Can you work these out from the model? Positions are in its coordinate system, mm. Give positions to 0.01 mm unless a question says otherwise; leave off trailing zeros. Write each loop counter-clockwise with the first axis right and the second up, starting at its lowest first coordinate (ties: lowest second). Pieces come first, ordered by that corner, then holes. Notation, with made-up numbers: (37, 82.5) -> (90, 82.5) arc R21 ccw to (90, 119.5) -> close; hole circle Ø7 at (13, 66.5). An arc over 180 degrees is marked (long way). Answer as CSV lines item,"result". Start each with the question number.
1. If we section it at D-D on x = 22.5: Write out the boundary of the cut face in (y, z).
2. I'm going to push flat-ended pins straight in: P1, Ø3, axis at x = 22.5, y = 5, coming from the +Z side; P2, Ø4, axis at x = 35.5, z = -129, coming from the -Y side; P3, Ø1.4, axis at x = 37, y = 6.5, coming from the -Z side; P4, Ø5.5, axis at x = 36, z = -75.5, coming from the +Y side. Where does each tip first touch, or does it pass through?
3. I need wall thicknesses on line 1 (X direction, y = 5.5, z = -110); line 2 (X direction, y = 2, z = -56); line 3 (Y direction, x = 7.5, z = -44). Which ranges of each line are inside material? Lowest first, please. Write a range as [from, to].
4. If we section it at C-C on y = 5: Count the separate pieces of the cut face and the enclosed holes in it, plus the area to 3 significant figures.
5. If we section it at A-A on z = -82: Write out the boundary of the cut face in (x, y).
6. If we section it at B-B on x = 12: Write out the boundary of the cut face in (y, z), plus the area to 3 significant figures.
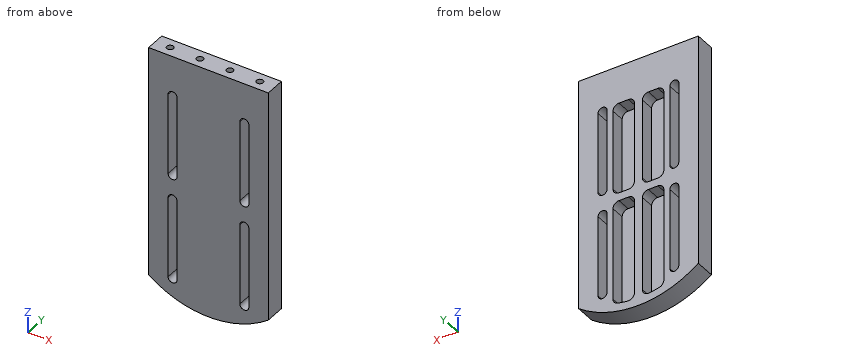
```python
from build123d import *

# Parameters (mm, degrees)
EXTRUDE_1_DEPTH     = 10
CUT_EXTRUDE_1_DEPTH = 7
EXTRUDE_2_REACH     = 173.532
SKETCH_3_W          = 10.75
SKETCH_3_H          = 4
FILLET_1_R          = 3
M4X0_71_D           = 3.3
M4X0_71_DEPTH       = 15
SKETCH_9_W          = 60
SKETCH_9_H          = 23.75
SKETCH_9_H_2        = 5
CUT_EXTRUDE_2_DEPTH = 10


with BuildPart() as part:
    # Эскиз1 → Бобышка-Вытянуть1 (new body)
    with BuildSketch(Plane(origin=(0, 0, 0), x_dir=(1, 0, 0), z_dir=(0, 1, 0))):
        with BuildLine():
            Line((0, 0), (0, 150.384470983))
            ThreePointArc((0, 150.384470983), (30, 160.384470983), (60, 150.384470983))
            Line((60, 150.384470983), (60, 0))
            Line((60, 0), (0, 0))
        make_face()
        with BuildLine():
            Line((14.25, 147.6), (14.25, 102))
            ThreePointArc((14.25, 102), (12, 99.75), (9.75, 102))
            Line((9.75, 102), (9.75, 147.6))
            ThreePointArc((9.75, 147.6), (12, 149.85), (14.25, 147.6))
        make_face(mode=Mode.SUBTRACT)
        with BuildLine():
            Line((50.25, 147.6), (50.25, 102))
            ThreePointArc((50.25, 102), (48, 99.75), (45.75, 102))
            Line((45.75, 102), (45.75, 147.6))
            ThreePointArc((45.75, 147.6), (48, 149.85), (50.25, 147.6))
        make_face(mode=Mode.SUBTRACT)
        with BuildLine():
            Line((14.25, 89.6), (14.25, 44))
            ThreePointArc((14.25, 44), (12, 41.75), (9.75, 44))
            Line((9.75, 44), (9.75, 89.6))
            ThreePointArc((9.75, 89.6), (12, 91.85), (14.25, 89.6))
        make_face(mode=Mode.SUBTRACT)
        with BuildLine():
            Line((45.75, 89.6), (45.75, 44))
            ThreePointArc((45.75, 44), (48, 41.75), (50.25, 44))
            Line((50.25, 44), (50.25, 89.6))
            ThreePointArc((50.25, 89.6), (48, 91.85), (45.75, 89.6))
        make_face(mode=Mode.SUBTRACT)
    extrude(amount=EXTRUDE_1_DEPTH)

    # Эскиз2 → Вырез-Вытянуть1 (cut)
    with BuildSketch(Plane(origin=(0, 10, 0), x_dir=(1, 0, 0), z_dir=(0, 1, 0))):
        with BuildLine():
            Line((4, 15), (28, 15))
            Line((28, 15), (28, 156.340972156))
            ThreePointArc((28, 156.340972156), (22.572755404, 155.780902976), (17.25, 154.5821802))
            Line((17.25, 154.5821802), (17.25, 44))
            ThreePointArc((17.25, 44), (15.712310601, 40.287689399), (12, 38.75))
            Line((12, 38.75), (4, 38.75))
            Line((4, 38.75), (4, 15))
        make_face()
        with BuildLine():
            Line((56, 15), (32, 15))
            Line((32, 15), (32, 156.340972156))
            ThreePointArc((32, 156.340972156), (37.427244596, 155.780902976), (42.75, 154.5821802))
            Line((42.75, 154.5821802), (42.75, 44))
            ThreePointArc((42.75, 44), (44.287689399, 40.287689399), (48, 38.75))
            Line((48, 38.75), (56, 38.75))
            Line((56, 38.75), (56, 15))
        make_face()
    extrude(amount=-CUT_EXTRUDE_1_DEPTH, mode=Mode.SUBTRACT)

    # Эскиз3 → Бобышка-Вытянуть2 (add, up to next)
    with BuildSketch(Plane(origin=(0, 10, 0), x_dir=(1, 0, 0), z_dir=(0, 1, 0)), mode=Mode.PRIVATE) as extrude_2_sk1:
        with BuildLine():
            ThreePointArc((17.099019514, 42.75), (15.240370349, 39.86932209), (12, 38.75))
            Line((12, 38.75), (28, 38.75))
            Line((28, 38.75), (28, 42.75))
            Line((28, 42.75), (17.099019514, 42.75))
        make_face()
    extrude_2_tool1 = extrude(extrude_2_sk1.sketch, amount=-EXTRUDE_2_REACH, mode=Mode.PRIVATE) - part.part
    # Эскиз3 → Бобышка-Вытянуть2 (add, up to next)
    with BuildSketch(Plane(origin=(0, 10, 0), x_dir=(1, 0, 0), z_dir=(0, 1, 0)), mode=Mode.PRIVATE) as extrude_2_sk2:
        with BuildLine():
            Line((32, 42.75), (32, 38.75))
            Line((32, 38.75), (48, 38.75))
            ThreePointArc((48, 38.75), (44.759629651, 39.86932209), (42.900980486, 42.75))
            Line((42.900980486, 42.75), (32, 42.75))
        make_face()
    extrude_2_tool2 = extrude(extrude_2_sk2.sketch, amount=-EXTRUDE_2_REACH, mode=Mode.PRIVATE) - part.part
    # Эскиз3 → Бобышка-Вытянуть2 (add, up to next)
    with BuildSketch(Plane(origin=(0, 10, 0), x_dir=(1, 0, 0), z_dir=(0, 1, 0)), mode=Mode.PRIVATE) as extrude_2_sk3:
        with Locations((22.625, 95.8)):
            Rectangle(SKETCH_3_W, SKETCH_3_H)
    extrude_2_tool3 = extrude(extrude_2_sk3.sketch, amount=-EXTRUDE_2_REACH, mode=Mode.PRIVATE) - part.part
    # Эскиз3 → Бобышка-Вытянуть2 (add, up to next)
    with BuildSketch(Plane(origin=(0, 10, 0), x_dir=(1, 0, 0), z_dir=(0, 1, 0)), mode=Mode.PRIVATE) as extrude_2_sk4:
        with Locations((37.375, 95.8)):
            Rectangle(SKETCH_3_W, SKETCH_3_H)
    extrude_2_tool4 = extrude(extrude_2_sk4.sketch, amount=-EXTRUDE_2_REACH, mode=Mode.PRIVATE) - part.part
    add(extrude_2_tool1.solids().sort_by_distance((21.839158, 10, -40.64687))[0])
    add(extrude_2_tool2.solids().sort_by_distance((38.160842, 10, -40.64687))[0])
    add(extrude_2_tool3.solids().sort_by_distance((22.625, 10, -95.8))[0])
    add(extrude_2_tool4.solids().sort_by_distance((37.375, 10, -95.8))[0])

    # Скругление1
    fillet_1_edges = [part.edges().sort_by_distance(p)[0] for p in [
        (32, 6.5, -38.75),
        (56, 6.5, -38.75),
        (56, 6.5, -15),
        (32, 6.5, -15),
        (4, 6.5, -15),
        (28, 6.5, -15),
        (28, 6.5, -38.75),
        (4, 6.5, -38.75),
        (17.25, 6.5, -93.8),
        (28, 6.5, -93.8),
        (17.099019514, 6.5, -42.75),
        (28, 6.5, -42.75),
        (32, 6.5, -42.75),
        (42.900980486, 6.5, -42.75),
        (42.75, 6.5, -93.8),
        (32, 6.5, -93.8),
        (32, 6.5, -156.340972156),
        (42.75, 6.5, -154.5821802),
        (42.75, 6.5, -97.8),
        (32, 6.5, -97.8),
        (17.25, 6.5, -97.8),
        (28, 6.5, -97.8),
        (17.25, 6.5, -154.5821802),
        (28, 6.5, -156.340972156),
    ]]
    fillet(fillet_1_edges, radius=FILLET_1_R)

    # Отверстие обработанное метчиком M4x0.71
    with Locations(Plane.XY):
        with Locations((7.5, 5), (22.5, 5), (37.5, 5), (52.5, 5)):
            Hole(M4X0_71_D / 2, depth=M4X0_71_DEPTH)

    # Эскиз9 → Вырез-Вытянуть2 (cut)
    with BuildSketch(Plane(origin=(0, 10, 0), x_dir=(1, 0, 0), z_dir=(0, 1, 0))):
        with Locations((30, 26.875)):
            Rectangle(SKETCH_9_W, SKETCH_9_H)
        with Locations((30, 74.766509245)):
            Rectangle(SKETCH_9_W, SKETCH_9_H_2)
        with Locations((30, 134.003959037)):
            Rectangle(SKETCH_9_W, SKETCH_9_H_2)
    extrude(amount=-CUT_EXTRUDE_2_DEPTH, mode=Mode.SUBTRACT)


with BuildPart() as cut_extrude_2_piece_1:
    # of the separate pieces the step leaves, piece 1, a body of its own (cut_extrude_2_pieces)
    add(part.part.solids().sort_by_distance((60, 10, -131.503959037))[0])


with BuildPart() as cut_extrude_2_piece_2:
    # of the separate pieces the step leaves, piece 2, a body of its own (cut_extrude_2_pieces)
    add(part.part.solids().sort_by_distance((60, 10, -72.266509245))[0])


with BuildPart() as cut_extrude_2_piece_3:
    # of the separate pieces the step leaves, piece 3, a body of its own (cut_extrude_2_pieces)
    add(part.part.solids().sort_by_distance((0, 10, 0))[0])


with BuildPart() as cut_extrude_2_piece_4:
    # of the separate pieces the step leaves, piece 4, a body of its own (cut_extrude_2_pieces)
    add(part.part.solids().sort_by_distance((60, 10, -150.384470983))[0])


with BuildPart() as cut_extrude_2_piece_1_1:
    # Move Body 1: read off the stored shape, not the designer's step
    # Move Body 1: moved
    add(cut_extrude_2_piece_1.part.moved(Location((0, 0, -5))))


with BuildPart() as cut_extrude_2_piece_2_1:
    # Move Body 2: read off the stored shape, not the designer's step
    # Move Body 2: moved
    add(cut_extrude_2_piece_2.part.moved(Location((0, 0, -10))))


with BuildPart() as cut_extrude_2_piece_3_1:
    # Move Body 3: read off the stored shape, not the designer's step
    # Move Body 3: moved
    add(cut_extrude_2_piece_3.part.moved(Location((0, 0, -33.75))))


with BuildPart() as cut_extrude_2_piece_4_1:
    add(cut_extrude_2_piece_4.part)

    # Combine 1: union Вырез-Вытянуть2 piece 1, Вырез-Вытянуть2 piece 2, Вырез-Вытянуть2 piece 3
    add(cut_extrude_2_piece_1_1.part)
    add(cut_extrude_2_piece_2_1.part)
    add(cut_extrude_2_piece_3_1.part)


solid = cut_extrude_2_piece_4_1.part
```
Computed values:
1,outline,"(0, -159.82) -> (10, -159.82) -> (10, -155.77) -> (3, -155.77) -> (3, -102.8) -> (10, -102.8) -> (10, -98.8) -> (3, -98.8) -> (3, -52.75) -> (10, -52.75) -> (10, -33.75) -> (6.65, -33.75) -> (6.65, -48.75) -> (3.35, -48.75) -> (3.35, -33.75) -> (0, -33.75) -> close"
2,P1,"stops at z = -48.75"
2,P2,"stops at y = 0"
2,P3,"stops at z = -159.99"
2,P4,"stops at y = 3"
3,line 1,"x = [0, 9.75], [14.25, 17.25], [28, 32], [42.75, 45.75], [50.25, 60]"
3,line 2,"x = [0, 9.75], [14.25, 45.75], [50.25, 60]"
3,line 3,"y = [0, 3.35], [6.65, 10]"
4,separate pieces,"1"
4,enclosed holes,"8"
4,area,"4,320 mm2"
5,outline,"(0, 0) -> (9.75, 0) -> (9.75, 10) -> (0, 10) -> close; (14.25, 0) -> (45.75, 0) -> (45.75, 10) -> (42.75, 10) -> (42.75, 3) -> (32, 3) -> (32, 10) -> (28, 10) -> (28, 3) -> (17.25, 3) -> (17.25, 10) -> (14.25, 10) -> close; (50.25, 0) -> (60, 0) -> (60, 10) -> (50.25, 10) -> close"
6,outline,"(0, -157.03) -> (10, -157.03) -> (10, -149.85) -> (0, -149.85) -> close; (0, -104.75) -> (10, -104.75) -> (10, -96.85) -> (0, -96.85) -> close; (0, -51.75) -> (10, -51.75) -> (10, -33.75) -> (0, -33.75) -> close"
6,area,"331 mm2"
